Could you check a few things on this drawing? It's one solid part, dimensions in mm from its lowest x, y, z. Coordinates: 2 decimals unless noted, no trailing zeros. Loops run counter-clockwise (first coordinate to the right, second up) from the corner with the lowest first, then second, coordinate; pieces in that order, holes last. Notation, with made-up numbers: (-19, 13.25) -> (0, 13.25) arc R26 ccw to (0, 35.25) -> close; hole circle Ø8 at (4.25, 28). An arc over 180 degrees is marked (long way). One line per question, with ' | ' between items.
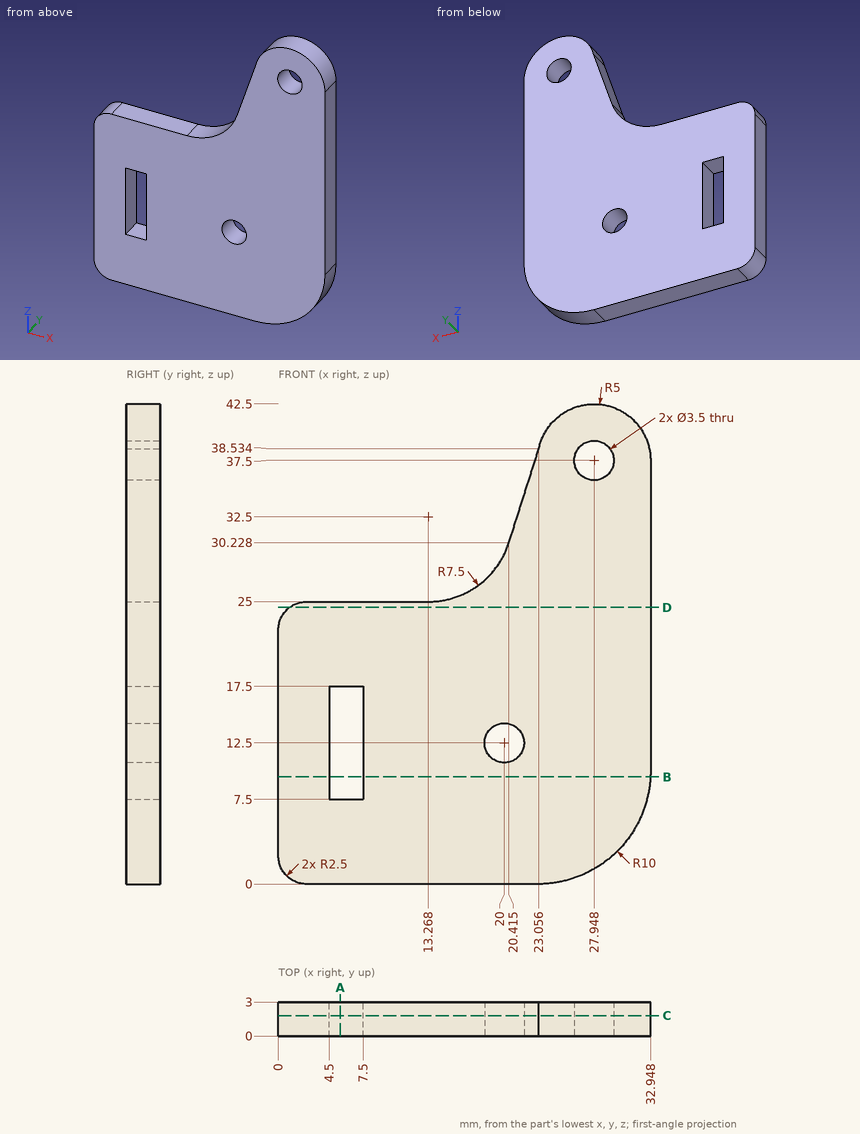
1) If we section it at D-D on z = 24.5: Please give me the cut outline in (x, y).
Data:
outline: (1, 0) -> (32.95, 0) -> (32.95, 3) -> (1, 3) -> close
2) If we section it at A-A on x = 5.5: Please give me the cut outline in (y, z).
Data:
outline: (0, 0) -> (3, 0) -> (3, 7.5) -> (0, 7.5) -> close; (0, 17.5) -> (3, 17.5) -> (3, 25) -> (0, 25) -> close
3) I need wall thicknesses on line 1 along X through (y, z) = (2.15, 12.5); line 2 along Z through (x, y) = (12, 0.6); line 3 along Z through (x, y) = (28.5, 0.45). Which ranges of each line are inside material? Lowest first, please. Write a range as from..to.
Data:
line 1: 0..4.5, 7.5..18.25, 21.75..32.95 | line 2: 0..25 | line 3: 1.68..35.84, 39.16..42.47
4) I'm going to push a flat-ended pin straight in: pin 1 Ø1.5 at (x, y) = (10.5, 2.5) entering from +Z. Where does the tip first touch, or does it pass through?
Data:
pin 1: z = 25
5) If we section it at B-B on z = 9.5: Please give me the cut outline in (x, y) (1 decimal).
Data:
outline: (0, 0) -> (4.5, 0) -> (4.5, 3) -> (0, 3) -> close; (7.5, 0) -> (32.9, 0) -> (32.9, 3) -> (7.5, 3) -> close
6) If we section it at C-C on y = 1.8: Give the number of separate pieces and of enclosed holes in the cut face, and give its area (3 significant figures).
Data:
separate pieces: 1 | enclosed holes: 3 | area: 948 mm²
